```python
from build123d import *

# Parameters (mm, degrees)
F0_W     = 500
F0_H     = 800
F0_R     = 7.5
F0_R_2   = 4.5
F1_DEPTH = 5
F3_DEPTH = 800
F5_DEPTH = 800.001


with BuildPart() as f1:
    # F0 (on Top) → F1 (new body)
    with BuildSketch(Plane.XY):
        with Locations((0, -175)):
            Rectangle(F0_W, F0_H)
        with Locations((-175, -461)):
            Circle(F0_R, mode=Mode.SUBTRACT)
        with Locations((175, -461)):
            Circle(F0_R, mode=Mode.SUBTRACT)
        with Locations((-217.5, 15)):
            Circle(F0_R_2, mode=Mode.SUBTRACT)
        with Locations((-132.5, 15)):
            Circle(F0_R_2, mode=Mode.SUBTRACT)
        with BuildLine():
            ThreePointArc((-200, 170), (-198.535534, 173.535534), (-195, 175))
            Line((-195, 175), (-155, 175))
            ThreePointArc((-155, 175), (-151.464466, 173.535534), (-150, 170))
            Line((-150, 170), (-150, -30))
            ThreePointArc((-150, -30), (-151.464466, -33.535534), (-155, -35))
            Line((-155, -35), (-195, -35))
            ThreePointArc((-195, -35), (-198.535534, -33.535534), (-200, -30))
            Line((-200, -30), (-200, 170))
        make_face(mode=Mode.SUBTRACT)
        with Locations((-217.5, 125)):
            Circle(F0_R_2, mode=Mode.SUBTRACT)
        with Locations((-132.5, 125)):
            Circle(F0_R_2, mode=Mode.SUBTRACT)
        with Locations((132.5, 15)):
            Circle(F0_R_2, mode=Mode.SUBTRACT)
        with Locations((217.5, 15)):
            Circle(F0_R_2, mode=Mode.SUBTRACT)
        with BuildLine():
            Line((195, -35), (155, -35))
            ThreePointArc((155, -35), (151.464466, -33.535534), (150, -30))
            Line((150, -30), (150, 170))
            ThreePointArc((150, 170), (151.464466, 173.535534), (155, 175))
            Line((155, 175), (195, 175))
            ThreePointArc((195, 175), (198.535534, 173.535534), (200, 170))
            Line((200, 170), (200, -30))
            ThreePointArc((200, -30), (198.535534, -33.535534), (195, -35))
        make_face(mode=Mode.SUBTRACT)
        with Locations((132.5, 125)):
            Circle(F0_R_2, mode=Mode.SUBTRACT)
        with Locations((217.5, 125)):
            Circle(F0_R_2, mode=Mode.SUBTRACT)
    extrude(amount=F1_DEPTH)

    # F2 (on face) → F3 (join, through all)
    with BuildSketch(Plane.XZ.offset(575)):
        with BuildLine():
            Line((25, 15), (0, 15))
            Line((0, 15), (-25, 15))
            ThreePointArc((-25, 15), (-28.535534, 13.535534), (-30, 10))
            Line((-30, 10), (-30, 5))
            Line((-30, 5), (30, 5))
            Line((30, 5), (30, 10))
            ThreePointArc((30, 10), (28.535534, 13.535534), (25, 15))
        make_face()
    extrude(amount=-F3_DEPTH)

    # F4 (on face) → F5 (cut, through all)
    with BuildSketch(Plane.XZ.offset(575)):
        with BuildLine():
            Line((-25, 5), (-25, 0))
            Line((-25, 0), (25, 0))
            Line((25, 0), (25, 5))
            ThreePointArc((25, 5), (23.535534, 8.535534), (20, 10))
            Line((20, 10), (-20, 10))
            ThreePointArc((-20, 10), (-23.535534, 8.535534), (-25, 5))
        make_face()
    extrude(amount=-F5_DEPTH, mode=Mode.SUBTRACT)


solid = f1.part
```
Part model, mm, in its own coordinate system. A direction names the side the tool comes from. Round coordinates to 2 decimals unless told otherwise and drop trailing zeros. Write each loop counter-clockwise with the first axis right and the second up, starting at its lowest first coordinate (ties: lowest second). Pieces come first, ordered by that corner, then holes. Notation, with made-up numbers: M 21,14.5 L 53,14.5 A32 ccw 53,40.5 Z; hole C -34.75,-22.5 d6. An arc over 180 degrees is marked long. Answer as CSV lines item,"result". Start each with the question number.
1) Band-saw the part on A-A (y = -315). List the corners of the cut face in (x, z), then the cut area to 3 significant figures.
2) Drop flat-ended pins along their axis: pin 1 (20 mm diameter, centred on x = 4.5, y = -255.5, fed in from -Z); pin 2 (12 mm diameter, centred on x = 109, y = -272.5, fed in from +Z); pin 3 (5 mm diameter, centred on y = 110, z = 8, fed in from -X). Give the stop position or say it passes through.
3) Band-saw the part on B-B (x = 72.5). List the corners of the cut face in (y, z).
4) Drill centre lines: L1, parallel to Y at x = 217.5, z = 3.85; L2, parallel to X at y = -461, z = 2; L3, parallel to Y at x = -175, z = 3.9. Where is each one in solid material? Low to high.
5) Mould opens along X. For faces 4 (the face through (-1.2, 225, 10.2)), 5 (the face through (0, -181, 10)) say: +X half, -X half, draft (parallel to the pull), parting line (faces both ways), or undercut.
6) Which spindle directions (+Z, -Z, +X, -X, +Y, -Y) get a long thin tool onto all of the face, cutting with end or side? Do faces 1 (the face through (-142, -169, 5)), 2 (the face through (138, -169, 5)), 3 (the face through (136, -169, 0)). Say none if no direction does.
Worked out:
1,outline,"M -250,0 L -25,0 L -25,5 A5 cw -20,10 L 20,10 A5 cw 25,5 L 25,0 L 250,0 L 250,5 L 30,5 L 30,10 A5 ccw 25,15 L -25,15 A5 ccw -30,10 L -30,5 L -250,5 Z"
1,area,"2,600 mm²"
2,pin 1,"z = 10"
2,pin 2,"z = 5"
2,pin 3,"x = -30"
3,outline,"M -575,0 L 225,0 L 225,5 L -575,5 Z"
4,L1,"-575 to 10.5, 19.5 to 120.5, 129.5 to 225"
4,L2,"-250 to -182.5, -167.5 to -25, 25 to 167.5, 182.5 to 250"
4,L3,"-575 to -468.5, -453.5 to -35, 175 to 225"
5,face 4,"draft"
5,face 5,"undercut"
6,face 1,"+Z, -X, +Y, -Y"
6,face 2,"+Z, +X, +Y, -Y"
6,face 3,"-Z, +X, -X, +Y, -Y"
